For this review, take the finished solid that the model builds, in its own axes (mm). Face numbers are marked on the shaded views. A direction names the side the tool comes from. Coordinates: 2 decimals unless noted, no trailing zeros. Loops run counter-clockwise (first coordinate to the right, second up) from the corner with the lowest first, then second, coordinate; pieces in that order, holes last. Notation, with made-up numbers: (61, -3.5) - (75, -3.5) arc R23 cw to (75, 12.5) - close; hole circle Ø6 at (48, -15). An arc over 180 degrees is marked (long way). Answer as a JSON object with one key per item and string values. Group by question number.
Item 1: We need section A-A (z = 2.1). Give the boundary of the cut face in (x, y) (3 decimals).
Item 2: Mouldability with a two-part tool opening along Y and no side actions: class the marked faces 3, 4 and 5 as released by +Y, released by -Y, zero draft, split by the parting line, or undercut.
Item 3: To check wall thickness, follow line 1 (Y direction, x = 0, z = 3.05); line 2 (Y direction, x = 1, z = 1.2); line 3 (X direction, y = -0.25, z = 2.6). State the ranges of each line that lie inside material, in increasing order.
Item 4: We need section B-B (x = 9). Give the boundary of the cut face in (y, z).
Item 5: We need section C-C (y = 12.25). Give the boundary of the cut face in (x, z).
Item 6: Tool access review of the marked faces 1 and 2: name each direction out of +Z, -Z, +X, -X, +Y, -Y from which nothing blocks a thin tool from reaching the whole face with its end or side.
Item 7: Clearance check with flat-ended pins moving along their axes: pin 1 (1.2 mm diameter, centred on x = 6, z = 2.5, fed in from +Y); pin 2 (1.5 mm diameter, centred on y = -2.5, z = 2.5, fed in from -X); pin 3 (1.5 mm diameter, centred on x = 26, z = 2.5, fed in from +Y). State where each tip first meets the part, or that it passes through.
from build123d import *

# Parameters (mm, degrees)
SKETCH1_R               = 1.5
BOSS_EXTRUDE3_DEPTH     = 4
CONG_3_R                = 1
CONG_4_R                = 1
ESQUISSE1_R             = 1.75
ENL_V_MAT_EXTRU_1_DEPTH = 10


with BuildPart() as part:
    # Sketch1 → Boss-Extrude3 (new body)
    with BuildSketch(Plane.XY):
        with BuildLine():
            Line((20.05, 5), (0, 5))
            ThreePointArc((0, 5), (-5, 0), (0, -5))
            Line((0, -5), (22, -5))
            Line((22, -5), (26.729403417, 1.622573056))
            Line((26.729403417, 1.622573056), (46.35880254, 9.735790053))
            Line((46.35880254, 9.735790053), (52.718761051, 7.224926885))
            Line((52.718761051, 7.224926885), (53.329707658, 6.286771643))
            Line((53.329707658, 6.286771643), (58.443335859, 8.389238381))
            Line((58.443335859, 8.389238381), (57.169030474, 11.488609151))
            Line((57.169030474, 11.488609151), (46.283795068, 15.786017162))
            Line((46.283795068, 15.786017162), (20.05, 5))
        make_face()
        Circle(SKETCH1_R, mode=Mode.SUBTRACT)
        with Locations((22.020705275, 0.206842568)):
            Circle(SKETCH1_R, mode=Mode.SUBTRACT)
    extrude(amount=BOSS_EXTRUDE3_DEPTH)

    # Congé3
    cong_3_edges = [part.edges().sort_by_distance(p)[0] for p in [
        (58.443335859, 8.389238381, 2),
        (53.329707658, 6.286771643, 2),
        (46.35880254, 9.735790053, 2),
    ]]
    fillet(cong_3_edges, radius=CONG_3_R)

    # Congé4
    cong_4_edges = [part.edges().sort_by_distance(p)[0] for p in [
        (46.283795068, 15.786017162, 2),
        (57.169030474, 11.488609151, 2),
    ]]
    fillet(cong_4_edges, radius=CONG_4_R)

    # Esquisse1 → Enlèv. mat.-Extru.1 (cut)
    with BuildSketch(Plane.XY.offset(4)):
        with Locations((22.020705275, 0.206842568)):
            Circle(ESQUISSE1_R)
        Circle(ESQUISSE1_R)
    extrude(amount=-ENL_V_MAT_EXTRU_1_DEPTH, mode=Mode.SUBTRACT)


solid = part.part
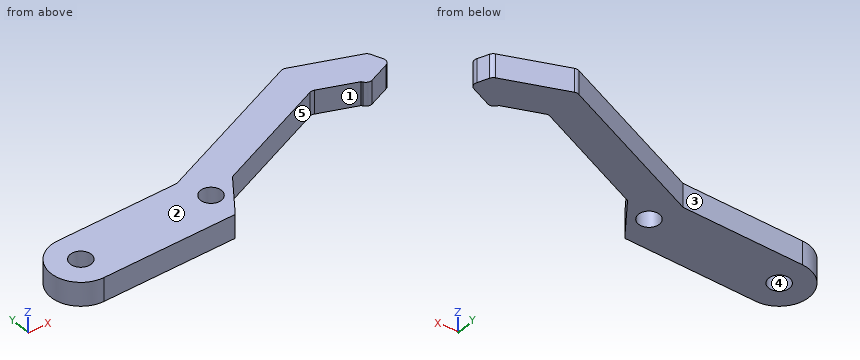
Check sheet entries:
{
 "1": {"outline": "(0, -5) - (22, -5) - (26.729, 1.623) - (45.985, 9.581) arc R1 cw to (46.735, 9.587) - (52.719, 7.225) - (52.878, 6.981) arc R1 ccw to (54.096, 6.602) - (57.518, 8.009) arc R1 ccw to (58.063, 9.314) - (57.331, 11.095) arc R1 ccw to (56.773, 11.645) - (46.659, 15.638) arc R1 ccw to (45.911, 15.633) - (20.05, 5) - (0, 5) arc R5 ccw to start; hole circle Ø3.5 at (0, 0); hole circle Ø3.5 at (22.021, 0.207)"},
 "2": {"face 3": "released by +Y", "face 4": "undercut", "face 5": "released by -Y"},
 "3": {"line 1": "y = -5 to -1.75, 1.75 to 5", "line 2": "y = -5 to -1.44, 1.44 to 5", "line 3": "x = -4.99 to -1.73, 1.73 to 20.33, 23.71 to 25.39"},
 "4": {"outline": "(-5, 0) - (5, 0) - (5, 4) - (-5, 4) - close"},
 "5": {"outline": "(37.68, 0) - (55.24, 0) - (55.24, 4) - (37.68, 4) - close"},
 "6": {"face 1": "+Z, -Z, -Y", "face 2": "+Z, +X, -X, +Y, -Y"},
 "7": {"pin 1": "stops at y = 5", "pin 2": "stops at x = -4.68", "pin 3": "stops at y = 7.75"}
}
